from build123d import *

# Parameters (mm, degrees)
BOSS_EXTRUDE1_DEPTH = 3.8
SKETCH3_R           = 0.9
BOSS_EXTRUDE2_DEPTH = 3
FILLET1_R           = 0.5
FILLET3_R           = 0.2


with BuildPart() as part:
    # Sketch2 → Boss-Extrude1 (new body)
    with BuildSketch(Plane.XY):
        with BuildLine():
            Line((-3.5, 0), (-2.55, 0))
            ThreePointArc((-2.55, 0), (0, 2.55), (2.55, 0))
            Line((2.55, 0), (3.5, 0))
            ThreePointArc((3.5, 0), (3.372684391, 0.935414347), (3, 1.802775638))
            Line((3, 1.802775638), (3, 2.5))
            ThreePointArc((3, 2.5), (2.707106781, 3.207106781), (2, 3.5))
            Line((2, 3.5), (0, 3.5))
            Line((0, 3.5), (-2, 3.5))
            ThreePointArc((-2, 3.5), (-2.707106781, 3.207106781), (-3, 2.5))
            Line((-3, 2.5), (-3, 1.802775638))
            ThreePointArc((-3, 1.802775638), (-3.372684391, 0.935414347), (-3.5, 0))
        make_face()
    extrude(amount=BOSS_EXTRUDE1_DEPTH)

    # Sketch3 → Boss-Extrude2 (add)
    with BuildSketch(Plane(origin=(0, 0, 0), x_dir=(1, 0, 0), z_dir=(0, 1, 0))):
        with Locations(Location((0, -1.9, 0), (0, 0, 90))):
            Circle(SKETCH3_R)
    extrude(amount=BOSS_EXTRUDE2_DEPTH)

    # Fillet1
    fillet1_edges = [part.edges().sort_by_distance(p)[0] for p in [
        (0, 0, 2.8),
    ]]
    fillet(fillet1_edges, radius=FILLET1_R)

    # Fillet3
    fillet3_edges = [part.edges().sort_by_distance(p)[0] for p in [
        (-3.025, 0, 3.8),
        (-3.025, 0, 0),
        (3.372684391, 0.935414347, 3.8),
        (3.372684391, 0.935414347, 0),
        (3.025, 0, 3.8),
        (3.5, 0, 1.9),
        (3.025, 0, 0),
        (0, 2.55, 2.8),
        (-2.55, 0, 1.9),
        (0, 2.55, 3.8),
        (2.55, 0, 1.9),
        (0, 2.55, 0),
        (-3, 2.151387819, 3.8),
        (-3, 2.151387819, 0),
        (-2.707106781, 3.207106781, 3.8),
        (-2.707106781, 3.207106781, 0),
        (0, 3.5, 3.8),
        (0, 3.5, 0),
        (2.707106781, 3.207106781, 3.8),
        (2.707106781, 3.207106781, 0),
        (3, 2.151387819, 3.8),
        (3, 2.151387819, 0),
        (-3.5, 0, 1.9),
        (3, 1.802775638, 1.9),
    ]]
    fillet(fillet3_edges, radius=FILLET3_R)


solid = part.part
Here's how the part is built. I have some questions about the finished solid (model axes, mm). Give positions to 0.01 mm unless a question says otherwise; leave off trailing zeros. Loops run counter-clockwise (first coordinate to the right, second up) from the corner with the lowest first, then second, coordinate; pieces in that order, holes last. Notation, with made-up numbers: (58, -40) -> (116, -40) arc R20 ccw to (116, -27) -> close; hole circle Ø3 at (30.5, -37.75). An arc over 180 degrees is marked (long way). One line per item, written item: value.
Q1. Suppose I cut it at B-B on y = 1.45. State how many separate pieces and enclosed holes the cut face has, then the cut area to 3 significant figures.
Answers follow:
separate pieces: 3
enclosed holes: 0
area: 10.8 mm^2
Q2. Suppose I cut it at A-A on z = 0.4. Please give me the cut outline in (x, y).
Answers follow:
outline: (-3.49, 0.21) arc R0.2 ccw to (-3.29, 0) -> (-2.74, 0) arc R0.2 ccw to (-2.54, 0.19) arc R2.55 cw to (2.54, 0.19) arc R0.2 ccw to (2.74, 0) -> (3.29, 0) arc R0.2 ccw to (3.49, 0.21) arc R3.5 ccw to (3.03, 1.76) arc R0.2 cw to (3, 1.86) -> (3, 2.5) arc R1 ccw to (2, 3.5) -> (-2, 3.5) arc R1 ccw to (-3, 2.5) -> (-3, 1.8) arc R3.5 ccw to start
Q3. We'd pull the mould along X, two halves only. Please class faces 1 (the face through (0.879, 1.412, 2.095)), 2 (the face through (0, 3.5, 2)), 3 (the face through (-2.699, 3.215, 1.876)): pulls with the +X half, pulls with the -X half, needs draft (parallel to the pull), parting line crosses it, or undercut.
Answers follow:
face 1: undercut
face 2: needs draft
face 3: pulls with the -X half
Q4. I'm going to push flat-ended pins straight in: pin 1 Ø1 at (x, z) = (1.5, 1) entering from -Y; pin 2 Ø2 at (y, z) = (3, 1) entering from +X; pin 3 Ø0.8 at (y, z) = (2.5, 2) entering from -X. Where does each tip first touch, or does it pass through?
Answers follow:
pin 1: y = 1.58
pin 2: x = 3
pin 3: x = -3
Q5. If I drill on line 1 along X through (y, z) = (1.55, 2.5); line 2 along X through (y, z) = (1.7, 1.2); line 3 along X through (y, z) = (2.55, 2.7), over which ranges is the centre line in solid material (lowest first)?
Answers follow:
line 1: -3.14 to -2.02, -0.67 to 0.67, 2.02 to 3.14
line 2: -3.06 to -1.9, -0.57 to 0.57, 1.9 to 3.06
line 3: -3 to 3
